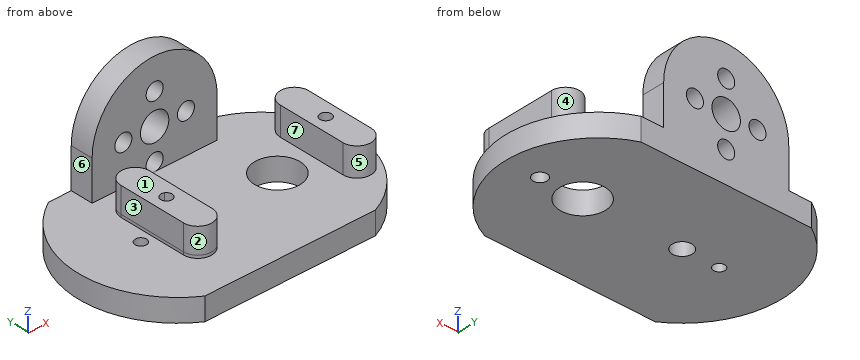
```python
from build123d import *

# Parameters (mm, degrees)
SKETCH1_R               = 1
SKETCH1_R_2             = 1.75
BOSS_EXTRUDE1_DEPTH     = 4
SKETCH2_R               = 1
BOSS_EXTRUDE2_DEPTH     = 5
CUT_EXTRUDE1_DEPTH      = 30.580398915
CUT_EXTRUDE1_DEPTH_BACK = 30.580398915
SKETCH2_3_R             = 4
SKETCH4_W               = 22
SKETCH4_H               = 4
BOSS_EXTRUDE3_DEPTH     = 22
FILLET1_RADIUS          = 11
FILLET1_LENGTH          = 4
SKETCH5_R               = 2.5
SKETCH5_R_2             = 1.5
CUT_EXTRUDE2_DEPTH      = 22
SKETCH8_R               = 1.25
CUT_EXTRUDE4_DEPTH      = 4
BOSS_EXTRUDE4_START     = -4.5
SKETCH11_R              = 1
BOSS_EXTRUDE4_DEPTH     = 4.5


with BuildPart() as part:
    # Sketch1 → Boss-Extrude1 (new body)
    with BuildSketch(Plane.XY):
        with BuildLine():
            Line((-15, 15), (15, 15))
            ThreePointArc((15, 15), (25, 0), (15, -15))
            Line((15, -15), (-15, -15))
            ThreePointArc((-15, -15), (-23.492855685, 0), (-15, 15))
        make_face()
        with Locations((12.5, 0)):
            Circle(SKETCH1_R, mode=Mode.SUBTRACT)
        with Locations((-6, 0)):
            Circle(SKETCH1_R_2, mode=Mode.SUBTRACT)
        with Locations((-12.5, 0)):
            Circle(SKETCH1_R, mode=Mode.SUBTRACT)
    extrude(amount=BOSS_EXTRUDE1_DEPTH)

    # Sketch2 → Boss-Extrude2 (add)
    # profile 1 of 2: a face of its own
    with BuildSketch(Plane.XY.offset(4)):
        with BuildLine():
            Line((22.50880699, -6), (22.50880699, 6))
            ThreePointArc((22.50880699, 6), (20.00880699, 8.5), (17.50880699, 6))
            Line((17.50880699, 6), (17.50880699, -6))
            ThreePointArc((17.50880699, -6), (20.00880699, -8.5), (22.50880699, -6))
        make_face()
        with Locations((20.00880699, 0)):
            Circle(SKETCH2_R, mode=Mode.SUBTRACT)
    # profile 2 of 2: a face of its own
    with BuildSketch(Plane.XY.offset(4)):
        with BuildLine():
            Line((-5.49119301, 1.674400026), (-5.49119301, 6))
            ThreePointArc((-5.49119301, 6), (-7.99119301, 8.5), (-10.49119301, 6))
            Line((-10.49119301, 6), (-10.49119301, -6))
            ThreePointArc((-10.49119301, -6), (-7.99119301, -8.5), (-5.49119301, -6))
            Line((-5.49119301, -6), (-5.49119301, -1.674400026))
            ThreePointArc((-5.49119301, -1.674400026), (-6.640863596, -1.628432944), (-7.5135021, -0.87852797))
            ThreePointArc((-7.5135021, -0.87852797), (-8.99119301, 0), (-7.5135021, 0.87852797))
            ThreePointArc((-7.5135021, 0.87852797), (-6.640863596, 1.628432944), (-5.49119301, 1.674400026))
        make_face()
    extrude(amount=BOSS_EXTRUDE2_DEPTH)

    # Sketch2<3> → Cut-Extrude1 (cut, two sides: drawn at the far end of the back side and taken through both)
    with BuildSketch(Plane.XY.offset(4).offset(-CUT_EXTRUDE1_DEPTH_BACK)):
        with Locations((11.50880699, 0)):
            Circle(SKETCH2_3_R)
    extrude(amount=CUT_EXTRUDE1_DEPTH + CUT_EXTRUDE1_DEPTH_BACK, mode=Mode.SUBTRACT)

    # Sketch4 → Boss-Extrude3 (add)
    with BuildSketch(Plane(origin=(0, 0, 0), x_dir=(-1, 0, 0), z_dir=(0, 0, -1))):
        with Locations((0, 13)):
            Rectangle(SKETCH4_W, SKETCH4_H)
    extrude(amount=-BOSS_EXTRUDE3_DEPTH)

    # Fillet1: full round fillet: the end face becomes a half cylinder, R = half its width
    fillet1_face = Plane((0, 13, 22), x_dir=(0, 1, 0), z_dir=(0, 0, 1))  # on the end face: x along it, z out of the body
    fillet1_slab = fillet1_face.offset(-FILLET1_RADIUS / 2) * Box(FILLET1_LENGTH, 2 * FILLET1_RADIUS, FILLET1_RADIUS, mode=Mode.PRIVATE)  # the body's end, R deep
    fillet1_round = Plane((0, 13, 11), x_dir=(0, 0, 1), z_dir=(0, 1, 0)) * Cylinder(FILLET1_RADIUS, FILLET1_LENGTH, mode=Mode.PRIVATE)  # its axis R under the face
    add(fillet1_slab - fillet1_round, mode=Mode.SUBTRACT)

    # Sketch5 → Cut-Extrude2 (cut)
    with BuildSketch(Plane(origin=(0, 15, 0), x_dir=(1, 0, 0), z_dir=(0, 1, 0))):
        with Locations(Location((0, -11, 0), (0, 0, 180))):
            Circle(SKETCH5_R)
        with Locations(Location((-5.5, -11, 0), (0, 0, 180))):
            Circle(SKETCH5_R_2)
        with Locations(Location((0, -5.5, 0), (0, 0, 180))):
            Circle(SKETCH5_R_2)
        with Locations(Location((5.5, -11, 0), (0, 0, 180))):
            Circle(SKETCH5_R_2)
        with Locations(Location((0, -16.5, 0), (0, 0, 180))):
            Circle(SKETCH5_R_2)
    extrude(amount=-CUT_EXTRUDE2_DEPTH, mode=Mode.SUBTRACT)

    # Sketch8 → Cut-Extrude4 (cut)
    with BuildSketch(Plane(origin=(0, 0, 0), x_dir=(-1, 0, 0), z_dir=(0, 0, -1))):
        with Locations((-19, 0)):
            Circle(SKETCH8_R)
    extrude(amount=-CUT_EXTRUDE4_DEPTH, mode=Mode.SUBTRACT)

    # Sketch11 → Boss-Extrude4 (add)
    with BuildSketch(Plane.XY.offset(9).offset(BOSS_EXTRUDE4_START)):
        with BuildLine():
            Line((-10.512429322, -6), (-10.512429322, 6))
            ThreePointArc((-10.512429322, 6), (-7.99119301, 8.521236312), (-5.469956698, 6))
            Line((-5.469956698, 6), (-5.469956698, -6))
            ThreePointArc((-5.469956698, -6), (-7.99119301, -8.521236312), (-10.512429322, -6))
        make_face()
        with Locations(Location((-7.99119301, 0, 0), (0, 0, 298.53470001))):
            Circle(SKETCH11_R, mode=Mode.SUBTRACT)
    extrude(amount=BOSS_EXTRUDE4_DEPTH)


solid = part.part
```
Part model, mm, in its own coordinate system. Face numbers are marked on the shaded views. A direction names the side the tool comes from. Coordinates: 2 decimals unless noted, no trailing zeros. Loops run counter-clockwise (first coordinate to the right, second up) from the corner with the lowest first, then second, coordinate; pieces in that order, holes last. Notation, with made-up numbers: (67.5, -20.75) - (91.5, -20.75) arc R30 ccw to (91.5, 2.25) - close; hole circle Ø6 at (57.5, -29). An arc over 180 degrees is marked (long way). Write item = value, one per line. Start each with the question number.
Item 1: Mould opens along X. For the marked faces 1, 2 and 3 say: released by +X, released by -X, zero draft, split by the parting line, or undercut.
Item 2: Flat gauge pins, fed straight in: pin 1 Ø5 at (x, z) = (0, 16.5) entering from -Y; pin 2 Ø5.5 at (x, y) = (-9, 3.5) entering from +Z; pin 3 Ø15 at (x, y) = (8.5, -1.5) entering from +Z; pin 4 Ø1.8 at (x, z) = (-5.5, 11) entering from -Y. Where does each tip first touch, or does it go through?
Item 3: 3-axis set-ups, long thin cutter, end or side, ignore diameter. For the marked faces 4, 5, 6 and 7: which of +Z, -Z, +X, -X, +Y, -Y reach the whole face in a straight line?
Item 4: Cut at B-B, the plane x = -12.5. Give the cut face in (y, z).
Item 5: Cut at A-A, the plane z = 5.5. Give the cut face in (x, y).
Item 6: Cut at C-C, the plane y = 11.5. Give the cut face in (x, z), and give its area (3 significant figures).
Item 7: Wall check: L1, parallel to Z at x = 0, y = 13.3; L2, parallel to X at y = -5.5, z = 4.25; L3, parallel to Y at x = -6, z = 1.65. Give the ranges that are in metal, low to high. Write a range as from..to.
The answers:
q1.face_1 = zero draft
q1.face_2 = undercut
q1.face_3 = released by -X
q2.pin_1 = 11
q2.pin_2 = 9
q2.pin_3 = 4
q2.pin_4 = through
q3.face_4 = +Z, +Y
q3.face_5 = +Z, -Y
q3.face_6 = +Z, -X, +Y, -Y
q3.face_7 = +Z, +Y, -Y
q4.outline = (-15, 0) - (-1, 0) - (-1, 4) - (-15, 4) - close; (1, 0) - (15, 0) - (15, 4) - (1, 4) - close
q5.outline = (-11, 11) - (-1.5, 11) - (-1.5, 15) - (-11, 15) - close; (-10.51, -6) arc R2.52 ccw to (-5.47, -6) - (-5.47, 6) arc R2.52 ccw to (-10.51, 6) - close; (1.5, 11) - (11, 11) - (11, 15) - (1.5, 15) - close; (17.51, -6) arc R2.5 ccw to (22.51, -6) - (22.51, 6) arc R2.5 ccw to (17.51, 6) - close; hole circle Ø2 at (-7.99, 0); hole circle Ø2 at (20.01, 0)
q6.outline = (-19.18, 0) - (20.23, 0) - (20.23, 4) - (11, 4) - (11, 11) arc R11 ccw to (-11, 11) - (-11, 4) - (-19.18, 4) - close; hole circle Ø3 at (-5.5, 11); hole circle Ø5 at (0, 11); hole circle Ø3 at (0, 5.5); hole circle Ø3 at (0, 16.5); hole circle Ø3 at (5.5, 11)
q6.area = 454 mm2
q7.L1 = 0..4, 7..8.5, 13.5..15, 18..22
q7.L2 = -10.49..-5.49, 17.51..22.51
q7.L3 = -15..-1.75, 1.75..15
